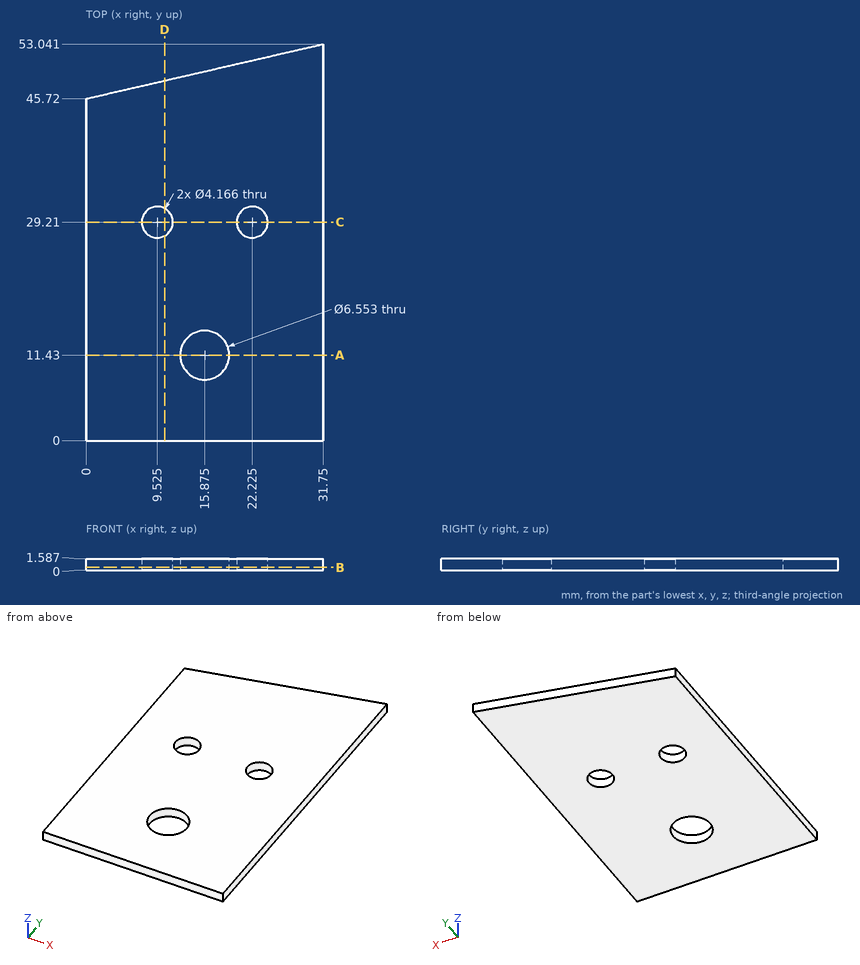
Input: dimensioned drawing with shaded views. Units: mm. Origin: part minimum x, y, z. Round coordinates to 2 decimals unless told otherwise and drop trailing zeros. Loops run counter-clockwise (first coordinate to the right, second up) from the corner with the lowest first, then second, coordinate; pieces in that order, holes last. Notation, with made-up numbers: M 46.25,-6.75 L 65.25,-6.75 A14 ccw 65.25,0.25 Z; hole C 3.5,9 d9. An arc over 180 degrees is marked long. Answer in a Markdown table with one row per item. Add a question column.
1. Section A-A (y = 11.43). Output: boundary loops of the cut face in (x, z).
2. Ray query, probe 1 along Y at (x, z) = (18, 0.55) (1 decimal); probe 2 along Y at (x, z) = (10.5, 0.35); probe 3 along X at (y, z) = (13, 0.65). Return the intervals inside material, ascending.
3. Section C-C (y = 29.21). Output: boundary loops of the cut face in (x, z).
4. Section D-D (x = 10.5). Output: boundary loops of the cut face in (y, z).
5. Contact query for a flat-ended pin moving along its axis: pin 1 (4 mm diameter, centred on x = 15.875, y = 11.43, fed in from +Z). Output: stop coordinate, or through.
6. Section B-B (z = 0.4). Give the number of separate pieces and of enclosed holes in the cut face, and give its area (3 significant figures).
Values follow:
| question | item | result |
|---|---|---|
| 1 | outline | M 0,0 L 12.6,0 L 12.6,1.59 L 0,1.59 Z; M 19.15,0 L 31.75,0 L 31.75,1.59 L 19.15,1.59 Z |
| 2 | probe 1 | 0 to 8.9, 13.9 to 49.9 |
| 2 | probe 2 | 0 to 27.37, 31.05 to 48.14 |
| 2 | probe 3 | 0 to 13, 18.75 to 31.75 |
| 3 | outline | M 0,0 L 7.44,0 L 7.44,1.59 L 0,1.59 Z; M 11.61,0 L 20.14,0 L 20.14,1.59 L 11.61,1.59 Z; M 24.31,0 L 31.75,0 L 31.75,1.59 L 24.31,1.59 Z |
| 4 | outline | M 0,0 L 27.37,0 L 27.37,1.59 L 0,1.59 Z; M 31.05,0 L 48.14,0 L 48.14,1.59 L 31.05,1.59 Z |
| 5 | pin 1 | through |
| 6 | separate pieces | 1 |
| 6 | enclosed holes | 3 |
| 6 | area | 1,510 mm^2 |
